```python
from build123d import *

# Parameters (mm, degrees)
BOSS_EXTRUDE1_DEPTH   = 3.175
F_6_CLEARANCE_HOLE1_D = 4.3053
SKETCH8_R             = 1.5875
SKETCH8_R_2           = 3.75
SKETCH8_R_3           = 6.4135
CUT_EXTRUDE1_DEPTH    = 4.175
F_6_CLEARANCE_HOLE2_D = 4.3053


with BuildPart() as part:
    # Sketch1 → Boss-Extrude1 (new body)
    with BuildSketch(Plane.XY):
        Polygon((0, 107.95), (0, 0), (63.5, 0), (63.5, 136.2202), align=None)
    extrude(amount=-BOSS_EXTRUDE1_DEPTH)

    # #6 Clearance Hole1 (through all)
    with Locations(Plane.XY):
        with Locations((58.6105, 14.2875), (4.8895, 14.2875), (4.8895, 90.4875), (58.6105, 109.5375)):
            Hole(F_6_CLEARANCE_HOLE1_D / 2)

    # Sketch8 → Cut-Extrude1 (cut, through all)
    with BuildSketch(Plane.XY):
        with Locations((20.373230618, 91.71042385)):
            Circle(SKETCH8_R)
        with Locations((47.270485986, 91.71042385)):
            Circle(SKETCH8_R)
        with Locations((47.270485986, 56.073006151)):
            Circle(SKETCH8_R)
        with Locations((32.1439032, 12.7)):
            Circle(SKETCH8_R_2)
        with Locations((20.373230618, 56.073006151)):
            Circle(SKETCH8_R)
        with Locations((32.1439032, 18.7)):
            Circle(SKETCH8_R)
        with Locations((47.270485986, 46.548006151)):
            Circle(SKETCH8_R_3)
        with Locations((47.270485986, 82.18542385)):
            Circle(SKETCH8_R_3)
        with Locations((20.373230618, 82.18542385)):
            Circle(SKETCH8_R_3)
        with Locations((20.373230618, 46.548006151)):
            Circle(SKETCH8_R_3)
    extrude(amount=-CUT_EXTRUDE1_DEPTH, mode=Mode.SUBTRACT)

    # #6 Clearance Hole2 (through all)
    with Locations(Plane(origin=(31.75, 0, 6.35), x_dir=(1, 0, 0), z_dir=(0, 0, 1))):
        with Locations((1.676331213, 81.383391323), (-13.818696068, 17.771227958)):
            Hole(F_6_CLEARANCE_HOLE2_D / 2)


solid = part.part
```
Can you work these out from the model? Positions are in its coordinate system, mm. Coordinates: 2 decimals unless noted, no trailing zeros.
Item 1: Suppose I cut it at A-A (z = -1.35). State how many separate pieces and enclosed holes the cut face has, then the cut area to 3 significant figures.
Answers below:
separate pieces: 1
enclosed holes: 16
area: 7,060 mm2
Item 2: Please list where these lines run through material, in increasing order: L1, parallel to Y at x = 20.5, z = -2.05; L2, parallel to X at y = 80.5, z = -2.8; L3, parallel to Y at x = 42.5, z = -1.
Answers below:
L1: y = 0 to 40.14, 52.96 to 54.49, 57.66 to 75.77, 88.6 to 90.13, 93.29 to 117.08
L2: x = 0 to 14.19, 26.56 to 31.46, 35.39 to 41.08, 53.46 to 63.5
L3: y = 0 to 42.26, 50.83 to 77.9, 86.47 to 126.87
Item 3: If we mould it in two halves opening along X, with no side actions, what happens to faces 1 (the face through (0, 55, -2)), 2 (the face through (31, 19.8, -1.6)), 3 (the face through (31, 54, 0)), 4 (the face through (63.5, 67, -2))? For each: released by +X, released by -X, zero draft, split by the parting line, or undercut.
Answers below:
face 1: released by -X
face 2: undercut
face 3: zero draft
face 4: released by +X
